from build123d import *

# Parameters (mm, degrees)
SKETCH_1_W          = 18
SKETCH_1_H          = 10
SKETCH_1_R          = 1.5
EXTRUDE_1_DEPTH     = 10
SKETCH_2_R          = 1.5
CUT_EXTRUDE_1_DEPTH = 10
SKETCH_4_R          = 1.5
CUT_EXTRUDE_2_DEPTH = 25


with BuildPart() as part:
    # 草图1 → 凸台-拉伸1 (new body)
    with BuildSketch(Plane(origin=(0, 0, 0), x_dir=(1, 0, 0), z_dir=(0, 1, 0))):
        Rectangle(SKETCH_1_W, SKETCH_1_H)
        with Locations(Location((-4, 0, 0), (0, 0, 270))):
            Circle(SKETCH_1_R, mode=Mode.SUBTRACT)
        with Locations(Location((4, 0, 0), (0, 0, 270))):
            Circle(SKETCH_1_R, mode=Mode.SUBTRACT)
    extrude(amount=EXTRUDE_1_DEPTH)

    # 草图2 → 切除-拉伸1 (cut)
    with BuildSketch(Plane.XY.offset(5)):
        with Locations((-4, 5)):
            Circle(SKETCH_2_R)
        with Locations((4, 5)):
            Circle(SKETCH_2_R)
    extrude(amount=-CUT_EXTRUDE_1_DEPTH, mode=Mode.SUBTRACT)

    # 草图4 → 切除-拉伸2 (cut)
    with BuildSketch(Plane.ZY.offset(9)):
        with Locations(Location((0, 5, 0), (0, 0, 315))):
            Circle(SKETCH_4_R)
    extrude(amount=-CUT_EXTRUDE_2_DEPTH, mode=Mode.SUBTRACT)


solid = part.part
Could you check a few things on this model? Use its own coordinates, in mm. Give positions to 0.01 mm unless a question says otherwise; leave off trailing zeros. Order: outer loops, then holes, each group sorted by start corner. A loop starts at its lowest first (then second) coordinate and runs counter-clockwise, first axis right, second up. Notation, with made-up numbers: (-0.5, -25) - (19.5, -25) arc R27 cw to (19.5, 4) - close; hole circle Ø4 at (69.25, 6.25). An arc over 180 degrees is marked (long way). One line per question, with ' | ' between items. Start each with the question number.
Item 1: I want a section at D-D on y = 8.75. Write out the boundary of the cut face in (x, z), then the cut area to 3 significant figures.
Item 2: I want a section at C-C on x = -4. Write out the boundary of the cut face in (y, z), then the cut area to 3 significant figures.
Item 3: I want a section at A-A on z = 0. Write out the boundary of the cut face in (x, y), then the cut area to 3 significant figures.
Item 4: Thinking about a two-plate mould opening in Y: for faces 1 (the flat face through (0, 5, 5)), 2 (the flat face through (0, 10, 0)), 3 (the cylindrical face through (-5.11, 6.01, 3.06)), 4 (the flat face through (0, 0, 0)), which applies, pulls with the +Y half, pulls with the -Y half, needs draft (parallel to the pull), parting line crosses it, or undercut?
Item 5: I need wall thicknesses on probe 1 along X at (y, z) = (5, 2.25); probe 2 along Z at (x, y) = (-1.1, 5); probe 3 along Y at (x, z) = (4, -2.8). Which ranges of each line are inside material? Lowest first, please. Write a range as [from, to].
Item 6: I want a section at B-B on y = 5. Write out the boundary of the cut face in (x, z).
Item 7: I'm going to push a flat-ended pin straight in: pin 1 Ø2.5 at (y, z) = (5, 0) entering from +X. Where does the tip first touch, or does it pass through?
Verdict:
1) outline: (-9, -5) - (9, -5) - (9, 5) - (-9, 5) - close; hole circle Ø3 at (-4, 0); hole circle Ø3 at (4, 0) | area: 166 mm^2
2) outline: (0, -5) - (3.5, -5) - (3.5, -1.5) - (0, -1.5) - close; (0, 1.5) - (3.5, 1.5) - (3.5, 5) - (0, 5) - close; (6.5, -5) - (10, -5) - (10, -1.5) - (6.5, -1.5) - close; (6.5, 1.5) - (10, 1.5) - (10, 5) - (6.5, 5) - close | area: 49.0 mm^2
3) outline: (-9, 0) - (-5.5, 0) - (-5.5, 3.5) - (-9, 3.5) - close; (-9, 6.5) - (-5.5, 6.5) - (-5.5, 10) - (-9, 10) - close; (-2.5, 0) - (2.5, 0) - (2.5, 3.5) - (-2.5, 3.5) - close; (-2.5, 6.5) - (2.5, 6.5) - (2.5, 10) - (-2.5, 10) - close; (5.5, 0) - (9, 0) - (9, 3.5) - (5.5, 3.5) - close; (5.5, 6.5) - (9, 6.5) - (9, 10) - (5.5, 10) - close | area: 84.0 mm^2
4) face 1: needs draft | face 2: pulls with the +Y half | face 3: undercut | face 4: pulls with the -Y half
5) probe 1: [-9, -5.5], [-2.5, 2.5], [5.5, 9] | probe 2: [-5, -1.5], [1.5, 5] | probe 3: [0, 3.5], [6.5, 10]
6) outline: (-9, -5) - (-5.5, -5) - (-5.5, -1.5) - (-9, -1.5) - close; (-9, 1.5) - (-5.5, 1.5) - (-5.5, 5) - (-9, 5) - close; (-2.5, -5) - (2.5, -5) - (2.5, -1.5) - (-2.5, -1.5) - close; (-2.5, 1.5) - (2.5, 1.5) - (2.5, 5) - (-2.5, 5) - close; (5.5, -5) - (9, -5) - (9, -1.5) - (5.5, -1.5) - close; (5.5, 1.5) - (9, 1.5) - (9, 5) - (5.5, 5) - close
7) pin 1: through
